Here's how the part is built. I have some questions about the finished solid (model axes, mm). A direction names the side the tool comes from. Give positions to 0.01 mm unless a question says otherwise; leave off trailing zeros. Write each loop counter-clockwise with the first axis right and the second up, starting at its lowest first coordinate (ties: lowest second). Pieces come first, ordered by that corner, then holes. Notation, with made-up numbers: (-12, 6.25) -> (-7, 6.25) arc R8 cw to (-7, 18.25) -> close; hole circle Ø1 at (13.5, 8). An arc over 180 degrees is marked (long way). Answer as CSV lines item,"result". Start each with the question number.
from build123d import *

# Parameters (mm, degrees)
BOSS_EXTRU_1_DEPTH      = 550
ESQUISSE2_W             = 590
ESQUISSE2_H             = 710
BOSS_EXTRU_2_DEPTH      = 25
ESQUISSE3_W             = 330
ESQUISSE3_H             = 110
BOSS_EXTRU_3_DEPTH      = 1
ESQUISSE4_W             = 260
ESQUISSE4_H             = 3
ENL_V_MAT_EXTRU_1_DEPTH = 3


with BuildPart() as part:
    # Esquisse1 → Boss.-Extru.1 (new body)
    with BuildSketch(Plane.XY):
        Polygon((-215, 0), (215, 0), (215, 80), (176.208064244, 300), (-176.208064244, 300), (-215, 80), align=None)
    extrude(amount=BOSS_EXTRU_1_DEPTH)

    # Esquisse2 → Boss.-Extru.2 (add)
    with BuildSketch(Plane(origin=(0, 300, 0), x_dir=(1, 0, 0), z_dir=(0, 1, 0))):
        with Locations((50, -225)):
            Rectangle(ESQUISSE2_W, ESQUISSE2_H)
    extrude(amount=BOSS_EXTRU_2_DEPTH)

    # Esquisse3 → Boss.-Extru.3 (add)
    with BuildSketch(Plane(origin=(0, 325, 0), x_dir=(1, 0, 0), z_dir=(0, 1, 0))):
        with Locations((-30, -250)):
            Rectangle(ESQUISSE3_W, ESQUISSE3_H)
    extrude(amount=BOSS_EXTRU_3_DEPTH)

    # Esquisse4 → Enlèv. mat.-Extru.1 (cut)
    with BuildSketch(Plane(origin=(0, 326, 0), x_dir=(1, 0, 0), z_dir=(0, 1, 0))):
        with Locations((-30, -250)):
            Rectangle(ESQUISSE4_W, ESQUISSE4_H)
    extrude(amount=-ENL_V_MAT_EXTRU_1_DEPTH, mode=Mode.SUBTRACT)


solid = part.part
Item 1: If I drill on line 1 (Z direction, x = 175.5, y = 218.5); line 2 (Y direction, x = -219, z = 175.5); line 3 (X direction, y = 29, z = 121), over which ranges is the centre line in solid material (lowest first)? Write a range as [from, to].
Item 2: If we section it at B-B (x = 190): Please give me the cut outline in (y, z).
Item 3: If we section it at C-C (x = -128.5): Please give me the cut outline in (y, z), and give its area (3 significant figures).
Item 4: I'm going to push flat-ended pins straight in: pin 1 (6 mm diameter, centred on x = -36.5, y = 85.5, fed in from -Z); pin 2 (6 mm diameter, centred on y = 222, z = 107.5, fed in from +X); pin 3 (0.5 mm diameter, centred on y = 325.5, z = 269, fed in from +X). Where does each tip first touch, or does it pass through?
Item 5: For faces 4 (the face through (-3, 152, 0)), 5 (the face through (195.876, 188.46, 271.15)), 6 (the face through (-3, 152, 550)), 7 (the face through (-215, 41, 271)), which set-ups out of +Z, -Z, +X, -X, +Y, -Y let a thin tool reach every point of the face, with its end or its side?
Item 6: If we section it at D-D (y = 24): Please give me the cut outline in (x, z), and give its area (4 significant figures).
Item 7: If we section it at A-A (z = 286): Please give me the cut outline in (x, y).
Item 8: We'd pull the mould along Y, two halves only. Please class faces 1 (the face through (-3, 0, 271)), 2 (the face through (177, 300, 141)), 3 (the face through (215, 39, 271)): released by +Y, released by -Y, zero draft, split by the parting line, or undercut.
Final values:
1,line 1,"[0, 550]"
1,line 2,"[300, 325]"
1,line 3,"[-215, 215]"
2,outline,"(0, 0) -> (221.78, 0) -> (221.78, 550) -> (0, 550) -> close; (300, -130) -> (325, -130) -> (325, 580) -> (300, 580) -> close"
3,outline,"(0, 0) -> (300, 0) -> (300, -130) -> (325, -130) -> (325, 195) -> (326, 195) -> (326, 248.5) -> (323, 248.5) -> (323, 251.5) -> (326, 251.5) -> (326, 305) -> (325, 305) -> (325, 580) -> (300, 580) -> (300, 550) -> (0, 550) -> close"
3,area,"183,000 mm2"
4,pin 1,"z = 0"
4,pin 2,"x = 190.49"
4,pin 3,"x = 135"
5,face 4,"-Z, +X, -X, -Y"
5,face 5,"+Z, -Z, +X"
5,face 6,"+Z, +X, -X, -Y"
5,face 7,"+Z, -Z, -X, -Y"
6,outline,"(-215, 0) -> (215, 0) -> (215, 550) -> (-215, 550) -> close"
6,area,"236,500 mm2"
7,outline,"(-245, 300) -> (-176.21, 300) -> (-215, 80) -> (-215, 0) -> (215, 0) -> (215, 80) -> (176.21, 300) -> (345, 300) -> (345, 325) -> (135, 325) -> (135, 326) -> (-195, 326) -> (-195, 325) -> (-245, 325) -> close"
8,face 1,"released by -Y"
8,face 2,"undercut"
8,face 3,"zero draft"
